The listing builds one solid part. Answer for the finished solid, in the listing's coordinates (mm). A direction names the side the tool comes from. Coordinates: 2 decimals unless noted, no trailing zeros. Loops run counter-clockwise (first coordinate to the right, second up) from the corner with the lowest first, then second, coordinate; pieces in that order, holes last. Notation, with made-up numbers: (62, 0) -> (81, 0) arc R16 ccw to (81, 27) -> close; hole circle Ø8 at (36.5, 56.5). An arc over 180 degrees is marked (long way). Answer in a Markdown table with one row per item.
```python
from build123d import *

# Parameters (mm, degrees)
SKETCH1_W               = 60
SKETCH1_H               = 45
BOSS_EXTRUDE1_DEPTH     = 20
SKETCH2_W               = 20
SKETCH2_H               = 45
BOSS_EXTRUDE2_DEPTH     = 10
MFGCHAMFER1_START       = 28.637824638
MFGCHAMFER1_2_OUTLINE_W = 36.5
MFGCHAMFER1_2_OUTLINE_H = 2.828427124
MFGCHAMFER1_2_DEPTH     = 2.362175362


with BuildPart() as part:
    # Sketch1 → Boss-Extrude1 (new body)
    with BuildSketch(Plane.XY):
        Rectangle(SKETCH1_W, SKETCH1_H)
    extrude(amount=BOSS_EXTRUDE1_DEPTH)

    # Sketch2 → Boss-Extrude2 (add)
    with BuildSketch(Plane.XY.offset(20)):
        with Locations((-20, 0)):
            Rectangle(SKETCH2_W, SKETCH2_H)
    extrude(amount=BOSS_EXTRUDE2_DEPTH)

    # MfgChamfer1: read off the stored shape, not the designer's step
    # MfgChamfer1 outline → MfgChamfer1 (revolve, cut)
    with BuildSketch(Plane(origin=(-6.5, 22.5, 0), x_dir=(1, 0, 0), z_dir=(0, -1, 0))):
        Polygon((0, 20), (0, 18), (2, 20), align=None)
    revolve(axis=Axis((-6.5, 22.5, 0), (0, 0, 1)), mode=Mode.SUBTRACT)

    # MfgChamfer1 2 outline → MfgChamfer1 2 (cut)
    with BuildSketch(Plane(origin=(0, 0, 0), x_dir=(1, 0, 0), z_dir=(0, 0.707106781186547, 0.707106781186548)).offset(MFGCHAMFER1_START)):
        with Locations((11.75, 1.767766953)):
            Rectangle(MFGCHAMFER1_2_OUTLINE_W, MFGCHAMFER1_2_OUTLINE_H)
    extrude(amount=MFGCHAMFER1_2_DEPTH, mode=Mode.SUBTRACT)


solid = part.part
```
Item 1: A cutting plane is placed at C-C, the plane z = 21. Determine the outline of the cut face in (x, y), plus the area to 3 significant figures.
Findings below:
| item | result |
|---|---|
| outline | (-30, -22.5) -> (-10, -22.5) -> (-10, 22.5) -> (-30, 22.5) -> close |
| area | 900 mm2 |
Item 2: Find the intervals of material crossed by probe 1 along X at (y, z) = (-2, 27.5); probe 2 along Z at (x, y) = (27.5, -6.5); probe 3 along Y at (x, z) = (8, 19.5), in increasing order.
Findings below:
| item | result |
|---|---|
| probe 1 | x = -30 to -10 |
| probe 2 | z = 0 to 20 |
| probe 3 | y = -22.5 to 21 |
Item 3: A cutting plane is placed at B-B, the plane x = -3. Determine the outline of the cut face in (y, z).
Findings below:
| item | result |
|---|---|
| outline | (-22.5, 0) -> (22.5, 0) -> (22.5, 18) -> (20.5, 20) -> (-22.5, 20) -> close |
Item 4: A flat-ended cylindrical pin translates along its axis: pin 1 Ø11 at (y, z) = (3, 24) entering from +X. Find the tip coordinate at first contact, or state that the pin passes through.
Findings below:
| item | result |
|---|---|
| pin 1 | stops at x = 30 |
Item 5: A tool of negligible diameter and unlimited length cuts with its end or side. For faces 1 (the face through (-10, 0, 25)), 2 (the face through (11.5, 21.5, 19)), 3 (the face through (0, 0, 0)), from which of +Z, -Z, +X, -X, +Y, -Y can it reach the whole face along a straight path? Write none if from no direction.
Findings below:
| item | result |
|---|---|
| face 1 | +Z, +X, +Y, -Y |
| face 2 | +Z, +X, +Y |
| face 3 | -Z, +X, -X, +Y, -Y |
Item 6: A cutting plane is placed at A-A, the plane y = 14. Determine the outline of the cut face in (x, z).
Findings below:
| item | result |
|---|---|
| outline | (-30, 0) -> (30, 0) -> (30, 20) -> (-10, 20) -> (-10, 30) -> (-30, 30) -> close |
